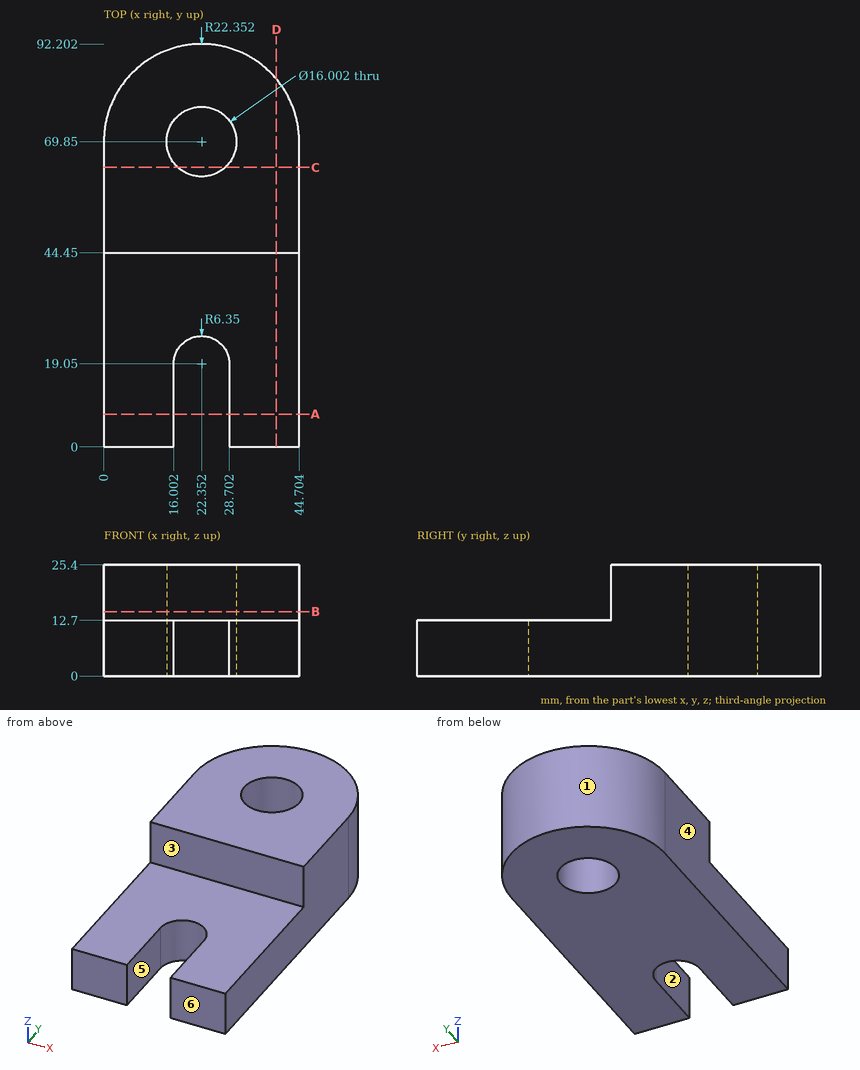
For this review, use the dimensioned drawing (mm, ordinates from the lowest corner) and the shaded views. A direction names the side the tool comes from. Round coordinates to 2 decimals unless told otherwise and drop trailing zeros. Write each loop counter-clockwise with the first axis right and the second up, starting at its lowest first coordinate (ties: lowest second). Pieces come first, ordered by that corner, then holes. Notation, with made-up numbers: (-6.75, 16) - (29.25, 16) arc R10 ccw to (29.25, 30) - close; hole circle Ø8 at (70, -7). An arc over 180 degrees is marked (long way). Use CSV: the item, a comma, the result in double quotes.
1) Add section A-A on y = 7.5. Write out the cut boundary in (x, z).
Conclusion:
outline,"(0, 0) - (16, 0) - (16, 12.7) - (0, 12.7) - close; (28.7, 0) - (44.7, 0) - (44.7, 12.7) - (28.7, 12.7) - close"
2) Clearance check with flat-ended pins moving along their axes: pin 1 Ø22 at (x, y) = (20.5, 21.5) entering from +Z; pin 2 Ø10 at (x, z) = (38.5, 21.5) entering from -Y; pin 3 Ø1.5 at (x, z) = (22, 13) entering from +Y. State where each tip first meets the part, or that it passes through.
Conclusion:
pin 1,"stops at z = 12.7"
pin 2,"stops at y = 44.45"
pin 3,"stops at y = 92.2"
3) Add section C-C on y = 64. Write out the cut boundary in (x, z), and give its area (3 significant figures).
Conclusion:
outline,"(0, 0) - (16.89, 0) - (16.89, 25.4) - (0, 25.4) - close; (27.81, 0) - (44.7, 0) - (44.7, 25.4) - (27.81, 25.4) - close"
area,"858 mm^2"
4) For the marked faces 1, 2 and 3, list the 3-axis set-ups (+Z, -Z, +X, -X, +Y, -Y) from which the entire face can be reached by the end or side of a thin tool; tool diameter is ignored.
Conclusion:
face 1,"+Z, -Z, +Y"
face 2,"+Z, -Z, -Y"
face 3,"+Z, +X, -X, -Y"
5) The part is to be moulded in two halves that separate along X. For the marked faces 4, 5 and 6, say which applies: pulls with the +X half, pulls with the -X half, needs draft (parallel to the pull), parting line crosses it, or undercut.
Conclusion:
face 4,"pulls with the -X half"
face 5,"undercut"
face 6,"needs draft"
6) Wall thickness on line 1 along Z through (x, y) = (35, 29); line 2 along Y through (x, z) = (27.5, 12); line 3 along Y through (x, z) = (23, 14.75): over which ranges is each line inside the solid? List them lowest first. Write a range as from..to.
Conclusion:
line 1,"z = 0..12.7"
line 2,"y = 22.77..63.73, 75.97..91.6"
line 3,"y = 44.45..61.88, 77.82..92.19"
7) Add section B-B on z = 14.75. Write out the cut boundary in (x, y), and give its area (3 significant figures).
Conclusion:
outline,"(0, 44.45) - (44.7, 44.45) - (44.7, 69.85) arc R22.35 ccw to (0, 69.85) - close; hole circle Ø16 at (22.35, 69.85)"
area,"1,720 mm^2"
8) Add section D-D on x = 39.5. Write out the cut boundary in (y, z).
Conclusion:
outline,"(0, 0) - (84.19, 0) - (84.19, 25.4) - (44.45, 25.4) - (44.45, 12.7) - (0, 12.7) - close"
